Model file for the job. Use its own axes, mm. Round coordinates to 2 decimals unless told otherwise and drop trailing zeros. Order: outer loops, then holes, each group sorted by start corner. A loop starts at its lowest first (then second) coordinate and runs counter-clockwise, first axis right, second up. Notation, with made-up numbers: (49.5, -0.5) - (101.5, -0.5) arc R22 cw to (101.5, 28.5) - close; hole circle Ø11 at (35, 46). An arc over 180 degrees is marked (long way). Use one line per item in the form item = value.
from build123d import *

# Parameters (mm, degrees)
F0_R     = 1.65
F0_R_2   = 2.55
F0_W     = 5
F0_H     = 10
F0_R_3   = 1.5
F0_R_4   = 3.555
F1_DEPTH = 4.75


# Not quite as in the source:
# - ends of sketch curves that miss each other by under 0.0002 mm in the source are joined


with BuildPart() as f1:
    # F0 (on Top) → F1 (new body)
    with BuildSketch(Plane.XY):
        with BuildLine():
            Line((-47.640397, 42.115595), (-100.031737, 108.050449))
            ThreePointArc((-100.031737, 108.050449), (-107.8442155419, 109.1246397394), (-109.2715048598, 101.368896092))
            Line((-109.2715048598, 101.368896092), (-54.999977, 18.664241))
            Line((-54.999977, 18.664241), (-54.999977, -18.664242))
            Line((-54.999977, -18.664242), (-109.271505, -101.368897))
            ThreePointArc((-109.271505, -101.368897), (-107.8441644553, -109.1246766812), (-100.031658534, -108.0503513703))
            Line((-100.031658534, -108.0503513703), (-47.643302, -42.116283))
            ThreePointArc((-47.643302, -42.116283), (-33.7130803066, -30.9767526972), (-16.325566, -27))
            Line((-16.325566, -27), (16.325565, -27))
            ThreePointArc((16.325565, -27), (33.7130793066, -30.9767526972), (47.6433013924, -42.1162826882))
            Line((47.6433013924, -42.1162826882), (100.031658, -108.050351))
            ThreePointArc((100.031658, -108.050351), (107.8441644255, -109.1246767027), (109.2715050175, -101.3688963323))
            Line((109.2715050175, -101.3688963323), (54.999976, -18.664242))
            Line((54.999976, -18.664242), (54.999976, 18.664241))
            Line((54.999976, 18.664241), (109.271504, 101.368896))
            ThreePointArc((109.271504, 101.368896), (107.8442155121, 109.1246397609), (100.0317360662, 108.0504489474))
            Line((100.0317360662, 108.0504489474), (47.640396, 42.115595))
            ThreePointArc((47.640396, 42.115595), (33.7103248028, 30.9765618002), (16.323206, 27))
            Line((16.323206, 27), (-16.323206, 27))
            ThreePointArc((-16.323206, 27), (-33.710325083, 30.9765619354), (-47.640397, 42.115595))
        make_face()
        with Locations((-104.5, -104.5)):
            Circle(F0_R, mode=Mode.SUBTRACT)
        with Locations((-44.444977, -20.807752)):
            Circle(F0_R_2, mode=Mode.SUBTRACT)
        with Locations((-49.499977, 0)):
            Rectangle(F0_W, F0_H, mode=Mode.SUBTRACT)
        with BuildLine():
            Line((-19.581953, -16.373154), (-39.803759, -2.743263))
            ThreePointArc((-39.803759, -2.743263), (-40.6136447533, -1.8442487652), (-40.906473, -0.670199))
            Line((-40.906473, -0.670199), (-40.906473, 0.670176))
            ThreePointArc((-40.906473, 0.670176), (-40.6136450793, 1.8442251525), (-39.8037598701, 2.7432388072))
            Line((-39.8037598701, 2.7432388072), (-19.581955, 16.373149))
            ThreePointArc((-19.581955, 16.373149), (-17.0106188475, 16.5072580793), (-15.684668, 14.300086))
            Line((-15.684668, 14.300086), (-15.684668, -14.30009))
            ThreePointArc((-15.684668, -14.30009), (-17.0106178687, -16.5072615586), (-19.581953, -16.373154))
        make_face(mode=Mode.SUBTRACT)
        with Locations((-10, -10)):
            Circle(F0_R_3, mode=Mode.SUBTRACT)
        with Locations((104.5, -104.5)):
            Circle(F0_R, mode=Mode.SUBTRACT)
        with Locations((10, -10)):
            Circle(F0_R_3, mode=Mode.SUBTRACT)
        with Locations((44.444976, -20.807752)):
            Circle(F0_R_2, mode=Mode.SUBTRACT)
        with BuildLine():
            Line((19.581954, 16.373149), (39.803759, 2.743239))
            ThreePointArc((39.803759, 2.743239), (40.6136440793, 1.8442251525), (40.906472, 0.670176))
            Line((40.906472, 0.670176), (40.906472, -0.670199))
            ThreePointArc((40.906472, -0.670199), (40.6136437533, -1.8442487652), (39.803757719, -2.7432625831))
            Line((39.803757719, -2.7432625831), (19.581952, -16.373154))
            ThreePointArc((19.581952, -16.373154), (17.0106168687, -16.5072615586), (15.684667, -14.30009))
            Line((15.684667, -14.30009), (15.684667, 14.300086))
            ThreePointArc((15.684667, 14.300086), (17.0106178475, 16.5072580793), (19.581954, 16.373149))
        make_face(mode=Mode.SUBTRACT)
        with Locations((49.499976, 0)):
            Rectangle(F0_W, F0_H, mode=Mode.SUBTRACT)
        with Locations((-44.444977, 20.810818)):
            Circle(F0_R_4, mode=Mode.SUBTRACT)
        with Locations((-10, 10)):
            Circle(F0_R_3, mode=Mode.SUBTRACT)
        with Locations((-104.5, 104.5)):
            Circle(F0_R, mode=Mode.SUBTRACT)
        with Locations((10, 10)):
            Circle(F0_R_3, mode=Mode.SUBTRACT)
        with Locations((44.444976, 20.810818)):
            Circle(F0_R_4, mode=Mode.SUBTRACT)
        with Locations((104.5, 104.5)):
            Circle(F0_R, mode=Mode.SUBTRACT)
    extrude(amount=F1_DEPTH)


solid = f1.part
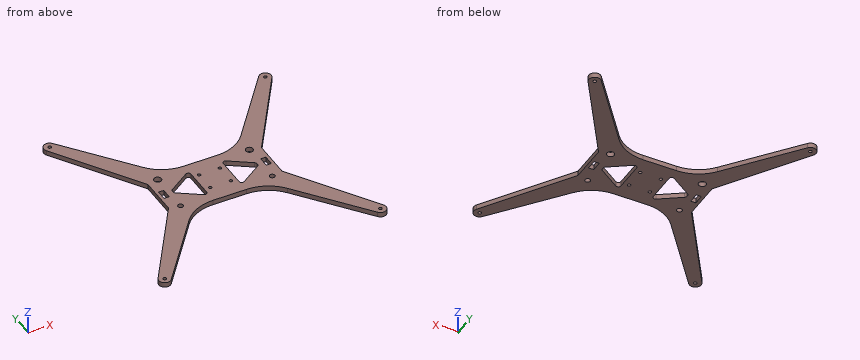
(1) Slice it at C-C on x = -1.5. Give the cut face in (y, z), then the cut area to 4 significant figures.
Report:
outline = (-27, 0) - (27, 0) - (27, 4.75) - (-27, 4.75) - close
area = 256.5 mm2
(2) Probe probe 1 along Y at (x, z) = (10, 3.7); probe 2 along Y at (x, z) = (104.5, 3.5); probe 3 along X at (y, z) = (13, 2.5). List the from-to ranges inside material, lowest first. Write a range as [from, to].
Report:
probe_1 = [-27, -11.5], [-8.5, 8.5], [11.5, 27]
probe_2 = [-110.21, -106.15], [-102.85, -94.1], [94.1, 102.85], [106.15, 110.21]
probe_3 = [-55, -24.59], [-15.68, 15.68], [24.59, 55]
(3) Slice it at B-B on x = 60. Give the cut face in (y, z), then the cut area to 3 significant figures.
Report:
outline = (-57.67, 0) - (-26.28, 0) - (-26.28, 4.75) - (-57.67, 4.75) - close; (26.28, 0) - (57.67, 0) - (57.67, 4.75) - (26.28, 4.75) - close
area = 298 mm2
(4) Slice it at A-A on y = 50. Give the cut face in (x, z).
Report:
outline = (-75.56, 0) - (-53.91, 0) - (-53.91, 4.75) - (-75.56, 4.75) - close; (53.91, 0) - (75.56, 0) - (75.56, 4.75) - (53.91, 4.75) - close
(5) Pin check, flat tips, straight feed: pin 1 (1.8 mm diameter, centred on x = -10, y = -10, fed in from +Z); pin 2 (5 mm diameter, centred on x = 10, y = -10, fed in from -Z); pin 3 (2.5 mm diameter, centred on y = -2, z = 3, fed in from -X); pin 4 (1 mm diameter, centred on x = 66, z = 1, fed in from -Y). Stop position of each tip, or through.
Report:
pin_1 = through
pin_2 = 0
pin_3 = -55
pin_4 = -65.85
(6) Slice it at D-D on z = 2.2. Count the separate pieces of the cut face and the enclosed holes in it, then the cut area to 3 significant figures.
Report:
separate_pieces = 1
enclosed_holes = 16
area = 11,200 mm2
